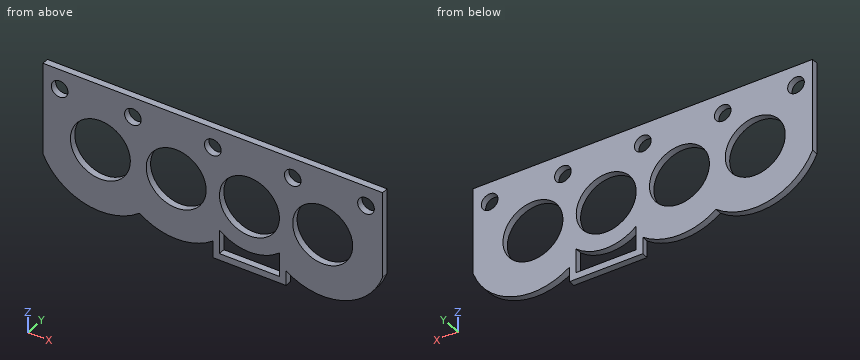
from build123d import *

# Parameters (mm, degrees)
SKETCH1_R           = 1.25
SKETCH1_R_2         = 4.5
BOSS_EXTRUDE1_DEPTH = 1


with BuildPart() as part:
    # Sketch1 → Boss-Extrude1 (new body)
    with BuildSketch(Plane(origin=(0, 0, 0), x_dir=(1, 0, 0), z_dir=(0, 1, 0))):
        with BuildLine():
            ThreePointArc((25.5, 17.461803162), (19.998907706, 19.269762955), (14.498241643, 17.46050678))
            ThreePointArc((14.498241643, 17.46050678), (6.411295647, 19.240430542), (0, 14))
            Line((0, 14), (0, 0))
            Line((0, 0), (51, 0))
            Line((51, 0), (51, 13.041381265))
            ThreePointArc((51, 13.041381265), (44.93185624, 19.036272406), (36.5, 17.745966692))
            Line((36.5, 17.745966692), (36.5, 20))
            Line((36.5, 20), (25.5, 20))
            Line((25.5, 20), (25.5, 17.461803162))
        make_face()
        with Locations(Location((48.5, 3, 0), (0, 0, 270))):
            Circle(SKETCH1_R, mode=Mode.SUBTRACT)
        with Locations(Location((37.5, 3, 0), (0, 0, 270))):
            Circle(SKETCH1_R, mode=Mode.SUBTRACT)
        with Locations(Location((25.5, 3, 0), (0, 0, 270))):
            Circle(SKETCH1_R, mode=Mode.SUBTRACT)
        with Locations(Location((8.61684397, 10, 0), (0, 0, 270))):
            Circle(SKETCH1_R_2, mode=Mode.SUBTRACT)
        with Locations(Location((20, 10, 0), (0, 0, 270))):
            Circle(SKETCH1_R_2, mode=Mode.SUBTRACT)
        with Locations(Location((31, 10, 0), (0, 0, 270))):
            Circle(SKETCH1_R_2, mode=Mode.SUBTRACT)
        with Locations(Location((42, 10, 0), (0, 0, 270))):
            Circle(SKETCH1_R_2, mode=Mode.SUBTRACT)
        with Locations(Location((2.5, 3, 0), (0, 0, 270))):
            Circle(SKETCH1_R, mode=Mode.SUBTRACT)
        with Locations(Location((13.5, 3, 0), (0, 0, 270))):
            Circle(SKETCH1_R, mode=Mode.SUBTRACT)
        with BuildLine():
            Line((35.5, 19), (35.5, 15.361902647))
            ThreePointArc((35.5, 15.361902647), (31, 17), (26.5, 15.361902647))
            Line((26.5, 15.361902647), (26.5, 19))
            Line((26.5, 19), (35.5, 19))
        make_face(mode=Mode.SUBTRACT)
    extrude(amount=BOSS_EXTRUDE1_DEPTH)


solid = part.part
Geometry check sheet. Reference: the model listing, model coordinates, mm. Coordinates: 2 decimals unless noted, no trailing zeros. Order: outer loops, then holes, each group sorted by start corner. A loop starts at its lowest first (then second) coordinate and runs counter-clockwise, first axis right, second up. Notation, with made-up numbers: (9.25, 3.25) - (40.25, 3.25) arc R33 cw to (40.25, 36.25) - close; hole circle Ø7 at (5.25, -1.5). An arc over 180 degrees is marked (long way). One line per item, written item: value.
(1) Sectioned sample at C-C (x = 42). Enter the section's corners in (y, z).
Data:
outline: (0, -19.5) - (1, -19.5) - (1, -14.5) - (0, -14.5) - close; (0, -5.5) - (1, -5.5) - (1, 0) - (0, 0) - close
(2) Sectioned sample at B-B (z = -3). Enter the section's corners in (x, y), and give its area (3 significant figures).
Data:
outline: (0, 0) - (1.25, 0) - (1.25, 1) - (0, 1) - close; (3.75, 0) - (12.25, 0) - (12.25, 1) - (3.75, 1) - close; (14.75, 0) - (24.25, 0) - (24.25, 1) - (14.75, 1) - close; (26.75, 0) - (36.25, 0) - (36.25, 1) - (26.75, 1) - close; (38.75, 0) - (47.25, 0) - (47.25, 1) - (38.75, 1) - close; (49.75, 0) - (51, 0) - (51, 1) - (49.75, 1) - close
area: 38.5 mm^2
(3) Sectioned sample at D-D (y = 0.2). Count the separate pieces of the cut face and the enclosed holes in it, and give its area (3 significant figures).
Data:
separate pieces: 1
enclosed holes: 10
area: 654 mm^2
(4) Thickness scan on probe 1 along X at (y, z) = (0.65, -10); probe 2 along X at (y, z) = (0.4, -3); probe 3 along X at (y, z) = (0.4, -13.25). Record the ranges inside material, lowest first. Write a range as from..to.
Data:
probe 1: x = 0..4.12, 13.12..15.5, 24.5..26.5, 35.5..37.5, 46.5..51
probe 2: x = 0..1.25, 3.75..12.25, 14.75..24.25, 26.75..36.25, 38.75..47.25, 49.75..51
probe 3: x = 0..5.5, 11.73..16.89, 23.11..27.89, 34.11..38.89, 45.11..50.93
(5) Sectioned sample at A-A (x = 31). Enter the section's corners in (y, z), and give its area (3 significant figures).
Data:
outline: (0, -20) - (1, -20) - (1, -19) - (0, -19) - close; (0, -17) - (1, -17) - (1, -14.5) - (0, -14.5) - close; (0, -5.5) - (1, -5.5) - (1, 0) - (0, 0) - close
area: 9.00 mm^2
